Build history of the part. All positions in model axes, mm. A direction names the side the tool comes from. Round coordinates to 2 decimals unless told otherwise and drop trailing zeros. Write each loop counter-clockwise with the first axis right and the second up, starting at its lowest first coordinate (ties: lowest second). Pieces come first, ordered by that corner, then holes.
Autodesk Fusion 360 part; units mm, degrees
sketch "Sketch1" plane through (0, 0, 0) normal (0, 0, 1) x (1, 0, 0)
  line L0 (10.9985, -6.35) -> (0, 12.7)
  line L1 (0, 12.7) -> (-10.9985, -6.35)
  line L2 (-10.9985, -6.35) -> (10.9985, -6.35)
  line L3 (3.6662, -6.35) -> (7.3323, 0) construction
  line L4 (7.3323, 0) -> (3.6662, 6.35) construction
  line L5 (3.6662, 6.35) -> (-3.6662, 6.35) construction
  line L6 (-3.6662, 6.35) -> (-7.3323, 0) construction
  line L7 (-7.3323, 0) -> (-3.6662, -6.35) construction
  line L8 (-3.6662, -6.35) -> (3.6662, -6.35) construction
  circle A0 centre (0, 0) radius 12.7
  arc A1 (3.2996, 6.985) -> (-3.2996, 6.985) centre (0, 5.08) ccw
  arc A2 (-7.699, -0.635) -> (-4.3994, -6.35) centre (-4.3994, -2.54) ccw
  arc A3 (4.3994, -6.35) -> (7.699, -0.635) centre (4.3994, -2.54) ccw
  dimension "d1" = 6.35
  dimension "d2" = 25.4
  dimension "d4" = 3.81
  dimension "d6" = 360
extrude "Extrude1" add sketch "Sketch1" along normal blind 12.7 contours L0 L2 A3 | L2 A0 | L0 A0 | L1 A0 | L1 L2 A2 | L0 L1 A1
sketch "Sketch2" plane through (0, 0, 0) normal (0, 1, 0) x (1, 0, 0)
  line L0 (0, -12.7) -> (0, -15.875)
  line L1 (-12.7, -12.7) -> (12.7, -12.7)
  line L2 (-12.7, 0) -> (12.7, 0)
  line L3 (12.7, -12.7) -> (12.7, -15.875)
  line L4 (0, -15.875) -> (12.7, -15.875)
  line L5 (0, 0) -> (0, -3.175) construction
  line L6 (0, -3.175) -> (0, -6.35) construction
  line L7 (0, -6.35) -> (0, -9.525) construction
  line L8 (0, -9.525) -> (0, -12.7) construction
  point P0 (0, -9.525)
  point P1 (0, -6.35)
  point P2 (0, -3.175)
  dimension "d9" = 3.175
  dimension "d10" = 12.7
revolve "Revolve1" add sketch "Sketch2" angle 360 about axis through (0, 0, 12.7) along (0, 0, 1)
sketch "Sketch3" plane through (0, 0, 15.875) normal (0, 0, 1) x (-1, 0, 0)
  circle A0 centre (0, 0) radius 12.7
  circle A1 centre (0, 0) radius 6.35
  dimension "d12" = 12.7
extrude "Extrude2" add sketch "Sketch3" along normal blind 25.4 contours A1
sketch "Sketch4" plane through (0, 0, 0) normal (1, 0, 0) x (0, 1, 0)
  line L0 (6.35, 41.275) -> (-6.35, 41.275)
  line L1 (-6.35, 15.875) -> (-6.35, 24.765) construction
  line L2 (-6.35, 24.765) -> (-4.826, 27.4046)
  line L3 (-4.826, 27.4046) -> (-4.826, 35.7866)
  line L4 (-4.826, 35.7866) -> (-6.35, 38.4263)
  line L5 (-6.35, 41.275) -> (-6.35, 38.4263) construction
  line L6 (-6.35, 38.4263) -> (-6.35, 24.765)
  line L7 (-6.35, 15.875) -> (6.35, 15.875)
  dimension "d15" = 8.89
  dimension "d16" = 8.382
  dimension "d17" = 150
  dimension "d18" = 150
  dimension "d19" = 1.524
extrude "Extrude3" cut sketch "Sketch4" along normal mid plane 12.7
hole "Hole1" at (0, 0, 9.525) at (0, 0, 3.175) direction (0, -1, 0) diameter 2.7686 depth 12.7 tip angle 180
pattern_circular "C-Pattern1" count 3 over 360 about axis through (0, 0, 0) along (0, 0, 1) of "Hole1"
equation "d7 = shankLength"
equation "d18 = d17"
equation "d20 = d12 / 2"
equation "shankLength = 0.5 in"
1) Slice it at A-A (x = 0). Write the cut outline in (y, z) (3 decimals).
Results:
outline: (-12.7, 0) - (-6.35, 0) - (-6.35, 1.791) - (-12.7, 1.791) - close; (-12.7, 4.559) - (-6.35, 4.559) - (-6.35, 8.141) - (-12.7, 8.141) - close; (-12.7, 10.909) - (-6.35, 10.909) - (-6.35, 12.7) - (8.89, 12.7) - (8.89, 0) - (12.7, 0) - (12.7, 15.875) - (6.35, 15.875) - (6.35, 41.275) - (-6.35, 41.275) - (-6.35, 38.426) - (-4.826, 35.787) - (-4.826, 27.405) - (-6.35, 24.765) - (-6.35, 15.875) - (-12.7, 15.875) - close
2) Slice it at D-D (y = 8.25). Write the cut outline in (x, z) (3 decimals).
Results:
outline: (-9.655, 0) - (-2.114, 0) - (-2.114, 12.7) - (2.114, 12.7) - (2.114, 0) - (9.655, 0) - (9.655, 15.875) - (-9.655, 15.875) - close
3) Slice it at B-B (y = -8). Write the cut outline in (x, z) (3 decimals), plus the area to 3 significant figures.
Results:
outline: (-9.864, 0) - (9.864, 0) - (9.864, 15.875) - (-9.864, 15.875) - close; hole circle Ø2.769 at (0, 3.175); hole circle Ø2.769 at (0, 9.525)
area: 301 mm2
4) Pin check, flat tips, straight feed: pin 1 Ø5 at (y, z) = (9, 32) entering from +X; pin 2 Ø1 at (x, z) = (0.5, 31) entering from +Y; pin 3 Ø8 at (y, z) = (-5.5, 11.5) entering from +X; pin 4 Ø2.5 at (x, z) = (2, 5) entering from +Y. Stop position of each tip, or through.
Results:
pin 1: passes through
pin 2: stops at y = 6.35
pin 3: stops at x = 12.61
pin 4: stops at y = 12.68
5) Which spindle directions (+Z, -Z, +X, -X, +Y, -Y) get a long thin tool onto all of the face, cutting with end or side? Do faces 1 (the flat face through (-0.058, -5.408, 36.795)), 2 (the cylindrical face through (0.53, -9.57, 10.804)), 3 (the cylindrical face through (-0.06, 8.89, 6.26)). Say none if no direction does.
Results:
face 1: +X, -X, -Y
face 2: -Y
face 3: -Z
6) Mould opens along X. For faces 4 (the flat face through (-0.06, -5.43, 26.36)), 5 (the cylindrical face through (0.8, 6.3, 28.4)), 6 (the flat face through (5.53, 3.12, 6.26)), 7 (the flat face through (-5.468, 3.228, 6.261)) say: released by +X, released by -X, zero draft, split by the parting line, or undercut.
Results:
face 4: zero draft
face 5: split by the parting line
face 6: undercut
face 7: undercut
7) Slice it at C-C (z = 28). Write the cut outline in (x, y).
Results:
outline: (-4.13, -4.83) - (4.13, -4.83) arc R6.35 ccw (long way) to start
8) Wall check: L1, parallel to Z at x = 0, y = -10.5 (3 decimals); L2, parallel to Z at x = 6.25, y = 5 (3 decimals); L3, parallel to Z at x = 5, y = 7.5 (3 decimals). Give the ranges that are in metal, low to high.
Results:
L1: z = 0 to 1.791, 4.559 to 8.141, 10.909 to 15.875
L2: z = 0 to 2.494, 3.856 to 8.844, 10.206 to 15.875
L3: z = 0 to 15.875
